Source: CAD feature listing. Evaluate the final solid. Frame: model axes, mm. Face numbers are marked on the shaded views. A direction names the side the tool comes from. Round coordinates to 2 decimals unless told otherwise and drop trailing zeros. Write each loop counter-clockwise with the first axis right and the second up, starting at its lowest first coordinate (ties: lowest second). Pieces come first, ordered by that corner, then holes. Notation, with made-up numbers: (-20.75, 45.25) -> (-13.75, 45.25) arc R20 ccw to (-13.75, 63.25) -> close; hole circle Ø10 at (16.25, -26). An arc over 180 degrees is marked (long way). Return JSON: item names as keys, results as strings. Group by question number.
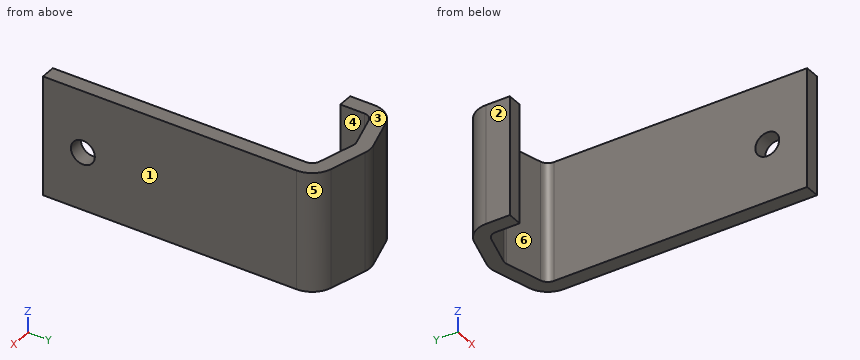
from build123d import *

# Parameters (mm, degrees)
F1_DEPTH = 25
F3_D     = 5


with BuildPart() as f1:
    # F0 (on Top) → F1 (new body)
    with BuildSketch(Plane.XY):
        with BuildLine():
            Line((-11.847499, 6.098918), (-11.847499, 1.069734))
            Line((-11.847499, 1.069734), (-8.747498, 1.069734))
            Line((-8.747498, 1.069734), (-8.747498, 6.098918))
            ThreePointArc((-8.747498, 6.098918), (-8.367381, 7.239074), (-7.379123, 7.923027))
            Line((-7.379123, 7.923027), (-0.488766, 9.931175))
            ThreePointArc((-0.488766, 9.931175), (0.027186, 10.007), (0.544318, 9.939697))
            Line((0.544318, 9.939697), (8.120311, 7.866691))
            ThreePointArc((8.120311, 7.866691), (9.129277, 7.186715), (9.518851, 6.03406))
            Line((9.518851, 6.03406), (9.518851, -46.987938))
            Line((9.518851, -46.987938), (12.618851, -46.987938))
            Line((12.618851, -46.987938), (12.618851, 6.03406))
            ThreePointArc((12.618851, 6.03406), (11.593656, 9.067363), (8.938482, 10.856775))
            Line((8.938482, 10.856775), (1.362489, 12.92978))
            ThreePointArc((1.362489, 12.92978), (0.001614, 13.106895), (-1.356153, 12.907354))
            Line((-1.356153, 12.907354), (-8.24651, 10.899206))
            ThreePointArc((-8.24651, 10.899206), (-10.84719, 9.099329), (-11.847499, 6.098918))
        make_face()
    extrude(amount=F1_DEPTH)

    # F3 (through all)
    with Locations(Plane(origin=(9.518851, 0, 0), x_dir=(0, -1, 0), z_dir=(-1, 0, 0))):
        with Locations((38.641255, 12.102515)):
            Hole(F3_D / 2)


solid = f1.part
Item 1: Set-up query: the marked faces 5 and 6. Return all of +Z, -Z, +X, -X, +Y, -Y with unobstructed straight access to the full face (end or side cutting, diameter ignored); none if empty.
Item 2: Cut plane B-B on z = 5.75. Output: boundary loops of the cut face in (x, y).
Item 3: Pull-direction query (X, two-part tool) for the marked faces 1, 2, 3 and 4; classes: +X half, -X half, draft (parallel to the pull), parting line (faces both ways), or undercut.
Item 4: Cut plane A-A on y = 5. Output: boundary loops of the cut face in (x, z), and give its area (3 significant figures).
Item 5: Material intervals for probe 1 along X at (y, z) = (2.5, 9.5); probe 2 along X at (y, z) = (-8, 7); probe 3 along Y at (x, z) = (10.75, 1.75), sorted ascending.
Item 6: First-contact query: pin 1 Ø4 at (x, z) = (-0.5, 21.5) entering from -Y (3 decimals); pin 2 Ø2.5 at (x, z) = (-10, 9.5) entering from -Y; pin 3 Ø6 at (y, z) = (-9.5, 8) entering from -X. Flat tips, straight axial feed; report the tip coordinate or a pass-through.
Item 7: Cut plane C-C on z = 10.25. Output: boundary loops of the cut face in (x, y).
Item 8: Cut plane D-D on x = -6. Output: boundary loops of the cut face in (y, z), and give its area (3 significant figures).
Here are the results:
{
 "1": {"face 5": "+Z, -Z, +X, +Y", "face 6": "+Z, -Z, -Y"},
 "2": {"outline": "(-11.85, 1.07) -> (-8.75, 1.07) -> (-8.75, 6.1) arc R1.9 cw to (-7.38, 7.92) -> (-0.49, 9.93) arc R1.9 cw to (0.54, 9.94) -> (8.12, 7.87) arc R1.9 cw to (9.52, 6.03) -> (9.52, -46.99) -> (12.62, -46.99) -> (12.62, 6.03) arc R5 ccw to (8.94, 10.86) -> (1.36, 12.93) arc R5 ccw to (-1.36, 12.91) -> (-8.25, 10.9) arc R5 ccw to (-11.85, 6.1) -> close"},
 "3": {"face 1": "+X half", "face 2": "-X half", "face 3": "draft", "face 4": "undercut"},
 "4": {"outline": "(-11.85, 0) -> (-8.75, 0) -> (-8.75, 25) -> (-11.85, 25) -> close; (9.52, 0) -> (12.62, 0) -> (12.62, 25) -> (9.52, 25) -> close", "area": "155 mm^2"},
 "5": {"probe 1": "x = -11.85 to -8.75, 9.52 to 12.62", "probe 2": "x = 9.52 to 12.62", "probe 3": "y = -46.99 to 9.93"},
 "6": {"pin 1": "stops at y = 9.345", "pin 2": "stops at y = 1.07", "pin 3": "stops at x = 9.52"},
 "7": {"outline": "(-11.85, 1.07) -> (-8.75, 1.07) -> (-8.75, 6.1) arc R1.9 cw to (-7.38, 7.92) -> (-0.49, 9.93) arc R1.9 cw to (0.54, 9.94) -> (8.12, 7.87) arc R1.9 cw to (9.52, 6.03) -> (9.52, -36.96) -> (12.62, -36.96) -> (12.62, 6.03) arc R5 ccw to (8.94, 10.86) -> (1.36, 12.93) arc R5 ccw to (-1.36, 12.91) -> (-8.25, 10.9) arc R5 ccw to (-11.85, 6.1) -> close; (9.52, -46.99) -> (12.62, -46.99) -> (12.62, -40.32) -> (9.52, -40.32) -> close"},
 "8": {"outline": "(8.32, 0) -> (11.55, 0) -> (11.55, 25) -> (8.32, 25) -> close", "area": "80.7 mm^2"}
}
